from build123d import *

# Parameters (mm, degrees)
F0_R     = 49.784
F1_DEPTH = 4.3561
F2_R     = 31.75
F3_DEPTH = 8.7132
F4_R     = 31.75
F5_DEPTH = 8.7132


with BuildPart() as f1:
    # F0 (on Front) → F1 (new body, symmetric)
    with BuildSketch(Plane.XZ):
        Circle(F0_R)
    extrude(amount=F1_DEPTH, both=True)

    # F2 (on face) → F3 (cut, through all)
    with BuildSketch(Plane.XZ.offset(4.3561)):
        Circle(F2_R)
    extrude(amount=-F3_DEPTH, mode=Mode.SUBTRACT)

    # F4 (on face) → F5 (intersect, through all)
    with BuildSketch(Plane.XZ.offset(4.3561)):
        with BuildLine():
            Line((-4.0281049428, 42.525724672), (-5.8042455242, 45.4699524537))
            ThreePointArc((-5.8042455242, 45.4699524537), (-6.9011720072, 46.9709680265), (-8.4606952501, 47.9829871535))
            ThreePointArc((-8.4606952501, 47.9829871535), (-9.5800368067, 46.4986118846), (-10.0974329669, 44.7129476743))
            Line((-10.0974329669, 44.7129476743), (-10.7594739569, 41.3388026977))
            ThreePointArc((-10.7594739569, 41.3388026977), (-13.8775459801, 38.1282442177), (-18.3298349378, 38.583416638))
            Line((-18.3298349378, 38.583416638), (-21.0058463435, 40.7426099021))
            ThreePointArc((-21.0058463435, 40.7426099021), (-22.5499976265, 41.7779322066), (-24.3616010367, 42.1955307493))
            ThreePointArc((-24.3616010367, 42.1955307493), (-24.9057517953, 40.4178369031), (-24.78121202, 38.5629015125))
            Line((-24.78121202, 38.5629015125), (-24.2493015044, 35.1658110223))
            ThreePointArc((-24.2493015044, 35.1658110223), (-26.0812551042, 31.0824294698), (-30.4207163198, 29.9873791269))
            Line((-30.4207163198, 29.9873791269), (-33.6738320805, 31.1011072995))
            ThreePointArc((-33.6738320805, 31.1011072995), (-35.4789607295, 31.5458611861), (-37.3241381993, 31.318670597))
            ThreePointArc((-37.3241381993, 31.318670597), (-37.2274655477, 29.4620742873), (-36.4760111717, 27.7616003006))
            Line((-36.4760111717, 27.7616003006), (-34.8143054089, 24.7513035456))
            ThreePointArc((-34.8143054089, 24.7513035456), (-35.1391799444, 20.287615), (-38.8424103517, 17.7744211264))
            Line((-38.8424103517, 17.7744211264), (-42.2802566958, 17.7083521531))
            ThreePointArc((-42.2802566958, 17.7083521531), (-44.1286375548, 17.5088937391), (-45.7848334494, 16.6643165564))
            ThreePointArc((-45.7848334494, 16.6643165564), (-45.0589975361, 14.9527506986), (-43.7712650475, 13.6118403748))
            Line((-43.7712650475, 13.6118403748), (-41.1801902767, 11.3514235709))
            ThreePointArc((-41.1801902767, 11.3514235709), (-39.9588010843, 7.0458147479), (-42.5791364422, 3.4176056157))
            Line((-42.5791364422, 3.4176056157), (-45.7870583635, 2.1797083896))
            ThreePointArc((-45.7870583635, 2.1797083896), (-47.4557494218, 1.3600953035), (-48.7232020734, 0))
            ThreePointArc((-48.7232020734, 0), (-47.4557494218, -1.3600953035), (-45.7870583635, -2.1797083896))
            Line((-45.7870583635, -2.1797083896), (-42.5791364422, -3.4176056157))
            ThreePointArc((-42.5791364422, -3.4176056157), (-39.9588010843, -7.0458147479), (-41.1801902767, -11.3514235709))
            Line((-41.1801902767, -11.3514235709), (-43.7712650475, -13.6118403748))
            ThreePointArc((-43.7712650475, -13.6118403748), (-45.0589975361, -14.9527506986), (-45.7848334494, -16.6643165564))
            ThreePointArc((-45.7848334494, -16.6643165564), (-44.1286375548, -17.5088937391), (-42.2802566958, -17.7083521531))
            Line((-42.2802566958, -17.7083521531), (-38.8424103517, -17.7744211264))
            ThreePointArc((-38.8424103517, -17.7744211264), (-35.1391799444, -20.287615), (-34.8143054089, -24.7513035456))
            Line((-34.8143054089, -24.7513035456), (-36.4760111717, -27.7616003006))
            ThreePointArc((-36.4760111717, -27.7616003006), (-37.2274655477, -29.4620742873), (-37.3241381993, -31.318670597))
            ThreePointArc((-37.3241381993, -31.318670597), (-35.4789607295, -31.5458611861), (-33.6738320805, -31.1011072995))
            Line((-33.6738320805, -31.1011072995), (-30.4207163198, -29.9873791269))
            ThreePointArc((-30.4207163198, -29.9873791269), (-26.0812551042, -31.0824294698), (-24.2493015044, -35.1658110223))
            Line((-24.2493015044, -35.1658110223), (-24.78121202, -38.5629015125))
            ThreePointArc((-24.78121202, -38.5629015125), (-24.9057517953, -40.4178369031), (-24.3616010367, -42.1955307493))
            ThreePointArc((-24.3616010367, -42.1955307493), (-22.5499976265, -41.7779322066), (-21.0058463435, -40.7426099021))
            Line((-21.0058463435, -40.7426099021), (-18.3298349378, -38.583416638))
            ThreePointArc((-18.3298349378, -38.583416638), (-13.8775459801, -38.1282442177), (-10.7594739569, -41.3388026977))
            Line((-10.7594739569, -41.3388026977), (-10.0974329669, -44.7129476743))
            ThreePointArc((-10.0974329669, -44.7129476743), (-9.5800368067, -46.4986118846), (-8.4606952501, -47.9829871535))
            ThreePointArc((-8.4606952501, -47.9829871535), (-6.9011720072, -46.9709680265), (-5.8042455242, -45.4699524537))
            Line((-5.8042455242, -45.4699524537), (-4.0281049428, -42.525724672))
            ThreePointArc((-4.0281049428, -42.525724672), (0, -40.57523), (4.0281049428, -42.525724672))
            Line((4.0281049428, -42.525724672), (5.8042455242, -45.4699524537))
            ThreePointArc((5.8042455242, -45.4699524537), (6.9011720072, -46.9709680265), (8.4606952501, -47.9829871535))
            ThreePointArc((8.4606952501, -47.9829871535), (9.5800368067, -46.4986118846), (10.0974329669, -44.7129476743))
            Line((10.0974329669, -44.7129476743), (10.7594739569, -41.3388026977))
            ThreePointArc((10.7594739569, -41.3388026977), (13.8775459801, -38.1282442177), (18.3298349378, -38.583416638))
            Line((18.3298349378, -38.583416638), (21.0058463435, -40.7426099021))
            ThreePointArc((21.0058463435, -40.7426099021), (22.5499976265, -41.7779322066), (24.3616010367, -42.1955307493))
            ThreePointArc((24.3616010367, -42.1955307493), (24.9057517953, -40.4178369031), (24.78121202, -38.5629015125))
            Line((24.78121202, -38.5629015125), (24.2493015044, -35.1658110223))
            ThreePointArc((24.2493015044, -35.1658110223), (26.0812551042, -31.0824294698), (30.4207163198, -29.9873791269))
            Line((30.4207163198, -29.9873791269), (33.6738320805, -31.1011072995))
            ThreePointArc((33.6738320805, -31.1011072995), (35.4789607295, -31.5458611861), (37.3241381993, -31.318670597))
            ThreePointArc((37.3241381993, -31.318670597), (37.2274655477, -29.4620742873), (36.4760111717, -27.7616003006))
            Line((36.4760111717, -27.7616003006), (34.8143054089, -24.7513035456))
            ThreePointArc((34.8143054089, -24.7513035456), (35.1391799444, -20.287615), (38.8424103517, -17.7744211264))
            Line((38.8424103517, -17.7744211264), (42.2802566958, -17.7083521531))
            ThreePointArc((42.2802566958, -17.7083521531), (44.1286375548, -17.5088937391), (45.7848334494, -16.6643165564))
            ThreePointArc((45.7848334494, -16.6643165564), (45.0589975361, -14.9527506986), (43.7712650475, -13.6118403748))
            Line((43.7712650475, -13.6118403748), (41.1801902767, -11.3514235709))
            ThreePointArc((41.1801902767, -11.3514235709), (39.9588010843, -7.0458147479), (42.5791364422, -3.4176056157))
            Line((42.5791364422, -3.4176056157), (45.7870583635, -2.1797083896))
            ThreePointArc((45.7870583635, -2.1797083896), (47.4557494218, -1.3600953035), (48.7232020734, 0))
            ThreePointArc((48.7232020734, 0), (47.4557494218, 1.3600953035), (45.7870583635, 2.1797083896))
            Line((45.7870583635, 2.1797083896), (42.5791364422, 3.4176056157))
            ThreePointArc((42.5791364422, 3.4176056157), (39.9588010843, 7.0458147479), (41.1801902767, 11.3514235709))
            Line((41.1801902767, 11.3514235709), (43.7712650475, 13.6118403748))
            ThreePointArc((43.7712650475, 13.6118403748), (45.0589975361, 14.9527506986), (45.7848334494, 16.6643165564))
            ThreePointArc((45.7848334494, 16.6643165564), (44.1286375548, 17.5088937391), (42.2802566958, 17.7083521531))
            Line((42.2802566958, 17.7083521531), (38.8424103517, 17.7744211264))
            ThreePointArc((38.8424103517, 17.7744211264), (35.1391799444, 20.287615), (34.8143054089, 24.7513035456))
            Line((34.8143054089, 24.7513035456), (36.4760111717, 27.7616003006))
            ThreePointArc((36.4760111717, 27.7616003006), (37.2274655477, 29.4620742873), (37.3241381993, 31.318670597))
            ThreePointArc((37.3241381993, 31.318670597), (35.4789607295, 31.5458611861), (33.6738320805, 31.1011072995))
            Line((33.6738320805, 31.1011072995), (30.4207163198, 29.9873791269))
            ThreePointArc((30.4207163198, 29.9873791269), (26.0812551042, 31.0824294698), (24.2493015044, 35.1658110223))
            Line((24.2493015044, 35.1658110223), (24.78121202, 38.5629015125))
            ThreePointArc((24.78121202, 38.5629015125), (24.9057517953, 40.4178369031), (24.3616010367, 42.1955307493))
            ThreePointArc((24.3616010367, 42.1955307493), (22.5499976265, 41.7779322066), (21.0058463435, 40.7426099021))
            Line((21.0058463435, 40.7426099021), (18.3298349378, 38.583416638))
            ThreePointArc((18.3298349378, 38.583416638), (13.8775459801, 38.1282442177), (10.7594739569, 41.3388026977))
            Line((10.7594739569, 41.3388026977), (10.0974329669, 44.7129476743))
            ThreePointArc((10.0974329669, 44.7129476743), (9.5800368067, 46.4986118846), (8.4606952501, 47.9829871535))
            ThreePointArc((8.4606952501, 47.9829871535), (6.9011720072, 46.9709680265), (5.8042455242, 45.4699524537))
            Line((5.8042455242, 45.4699524537), (4.0281049428, 42.525724672))
            ThreePointArc((4.0281049428, 42.525724672), (0, 40.57523), (-4.0281049428, 42.525724672))
        make_face()
        Circle(F4_R, mode=Mode.SUBTRACT)
    extrude(amount=-F5_DEPTH, mode=Mode.INTERSECT)


solid = f1.part
CAD build for the part. Positions are in the model's coordinates, mm. A direction names the side the tool comes from. Round coordinates to 2 decimals unless told otherwise and drop trailing zeros. Write each loop counter-clockwise with the first axis right and the second up, starting at its lowest first coordinate (ties: lowest second). Pieces come first, ordered by that corner, then holes. Notation, with made-up numbers: M -40,69 L 13,69 A27 cw 13,97 Z; hole C -1.75,-37 d2. An arc over 180 degrees is marked long. Put each result on its own line as item: value. Start each with the question number.
1) 3-axis set-ups, long thin cutter, end or side, ignore diameter. For faces 4 (the flat face through (-42.46, -0.06, -12.47)), 5 (the flat face through (32.025, -0.061, -30.536)), 6 (the flat face through (24.52, -0.06, -36.89)), 7 (the flat face through (32.07, -0.06, 30.55)): which of +Z, -Z, +X, -X, +Y, -Y reach the whole face in a straight line?
2) Pin check, flat tips, straight feed: pin 1 Ø2 at (x, y) = (-29, -0.5) entering from -Z; pin 2 Ø4 at (x, y) = (23, 3) entering from -Z; pin 3 Ø2 at (y, z) = (-2, 9.5) entering from -X. Stop position of each tip, or through.
3) Drill centre lines: probe 1 along Z at (x, y) = (0, 0.75); probe 2 along Z at (x, y) = (45.5, 3.75); probe 3 along Z at (x, y) = (14, -2.25). Where is each one in solid material? Low to high. Write a range as [from, to].
4) Saw through at A-A, the plane x = 0. Write the cut outline in (y, z), and give its area (3 significant figures).
5) Saw through at B-B, the plane x = 28. Write the cut outline in (y, z), and give its area (3 significant figures).
6) Pull direction X, two halves, no side cores. Call faces 1 (the cylindrical face through (-13.82, -0.06, 38.15)), 2 (the cylindrical face through (9.57, -0.06, -46.52)), 3 (the flat face through (-35.634, -0.061, -26.235)): pulls with the +X half, pulls with the -X half, needs draft (parallel to the pull), parting line crosses it, or undercut.
Resolved:
1. face 4: -X, +Y, -Y
1. face 5: -Z, +Y, -Y
1. face 6: +X, +Y, -Y
1. face 7: +Z, +Y, -Y
2. pin 1: z = -30.07
2. pin 2: z = -42.2
2. pin 3: x = -40.57
3. probe 1: [-40.58, -31.75], [31.75, 40.58]
3. probe 2: [-16.87, -15.78], [-2.29, 2.29], [15.78, 16.87]
3. probe 3: [-38.09, -28.5], [28.5, 38.09]
4. outline: M -4.36,-40.58 L 4.36,-40.58 L 4.36,-31.75 L -4.36,-31.75 Z; M -4.36,31.75 L 4.36,31.75 L 4.36,40.58 L -4.36,40.58 Z
4. area: 154 mm²
5. outline: M -4.36,-30.07 L 4.36,-30.07 L 4.36,-14.97 L -4.36,-14.97 Z; M -4.36,14.97 L 4.36,14.97 L 4.36,30.07 L -4.36,30.07 Z
5. area: 263 mm²
6. face 1: undercut
6. face 2: pulls with the +X half
6. face 3: pulls with the -X half
